Geometry check sheet. Reference: the model listing, model coordinates, mm. Face numbers are marked on the shaded views. A direction names the side the tool comes from. Give positions to 0.01 mm unless a question says otherwise; leave off trailing zeros. Loops run counter-clockwise (first coordinate to the right, second up) from the corner with the lowest first, then second, coordinate; pieces in that order, holes last. Notation, with made-up numbers: (7.25, 55.5) -> (21.25, 55.5) arc R27 cw to (21.25, 89.5) -> close; hole circle Ø6 at (57.25, 34.25). An arc over 180 degrees is marked (long way). Write each question's results on one line, items separated by ' | '. Start each with the question number.
1) Draft check along Z on the marked faces 1, 2 and 3. Enter one of: pulls with the +Z half, pulls with the -Z half, needs draft (parallel to the pull), parting line crosses it, or undercut.
2) Scan lines: line 1 (Z direction, x = 0.6, y = 0); line 2 (Z direction, x = -11.5, y = -7.5); line 3 (Y direction, x = -6, z = 7.25). Record each from-to range of solid material in increasing order. Write a range as from..to.
3) Set-up check for the marked faces 4, 5 and 6: record each of +Z, -Z, +X, -X, +Y, -Y from which the full face is reachable in a straight line by a thin tool's end or side.
4) Depth check by flat-ended pin: pin 1 (3 mm diameter, centred on x = -8, z = -6, fed in from +Y); pin 2 (12 mm diameter, centred on x = -2.5, y = 1.5, fed in from +Z); pin 3 (7.5 mm diameter, centred on x = -14.5, y = 3.5, fed in from -Z); pin 4 (7.5 mm diameter, centred on x = -13.5, y = 1.5, fed in from +Z). Enter the tip coordinate at first touch or a pass-through.
5) Sectioned sample at B-B on x = -12.5. Record the cut outline in (y, z), then the cut area to 3 significant figures.
6) Sectioned sample at D-D on x = -19. Record the cut outline in (y, z), then the cut area to 3 significant figures.
7) Sectioned sample at C-C on x = 6.5. Record the cut outline in (y, z), then the cut area to 3 significant figures.
8) Sectioned sample at A-A on z = 0. Record the cut outline in (x, y).
```python
from build123d import *

# Parameters (mm, degrees)
CROQUIS1_ONE_SIDE_W     = 3.003658151
CROQUIS1_ONE_SIDE_H     = 0.614983514
CROQUIS2_W              = 2.5
CROQUIS2_H              = 25
SALIENTE_EXTRUIR1_DEPTH = 25
CORTAR_EXTRUIR1_DEPTH   = 25


with BuildPart() as part:
    # Croquis1 one side → Revolución1 (revolve)
    with BuildSketch(Plane.XY, mode=Mode.PRIVATE) as revoluci_n1_sk:
        Polygon((-3.75, 15), (-3.75, 0), (3.75, 0), (8.75, 0), (8.75, 5), (3.75, 5), (3.75, 15), (1.503658151, 15), (0.751829076, 13.697793843), (-0.751829076, 13.697793843), (-1.503658151, 15), align=None)
        with Locations((0.001829075, 4.692508243)):
            Rectangle(CROQUIS1_ONE_SIDE_W, CROQUIS1_ONE_SIDE_H, mode=Mode.SUBTRACT)
    revolve(revoluci_n1_sk.sketch.rotate(Axis((-10.104371621, 0, 0), (1, 0, 0)), 180), axis=Axis((-10.104371621, 0, 0), (1, 0, 0)))

    # Croquis2 → Saliente-Extruir1 (add)
    with BuildSketch(Plane.ZY.offset(3.75)):
        with Locations((-6.75, 0)):
            Rectangle(CROQUIS2_W, CROQUIS2_H)
        with Locations((6.75, 0)):
            Rectangle(CROQUIS2_W, CROQUIS2_H)
    extrude(amount=SALIENTE_EXTRUIR1_DEPTH)

    # Croquis3 → Cortar-Extruir1 (cut)
    with BuildSketch(Plane.XY.offset(8)):
        with BuildLine():
            Line((-16.469719797, 12.5), (-28.75, 12.5))
            Line((-28.75, 12.5), (-28.75, 0.219719797))
            ThreePointArc((-28.75, 0.219719797), (-25.090200133, 8.840200133), (-16.469719797, 12.5))
        make_face()
        with BuildLine():
            Line((-28.75, -0.219719797), (-28.75, -12.5))
            Line((-28.75, -12.5), (-16.469719797, -12.5))
            ThreePointArc((-16.469719797, -12.5), (-25.090200133, -8.840200133), (-28.75, -0.219719797))
        make_face()
        with BuildLine():
            ThreePointArc((-11.25, 0), (-12.714466094, 3.535533906), (-16.25, 5))
            Line((-16.25, 5), (-16.25, -5))
            ThreePointArc((-16.25, -5), (-12.714466094, -3.535533906), (-11.25, 0))
        make_face()
        with BuildLine():
            Line((-16.25, -5), (-16.25, 5))
            ThreePointArc((-16.25, 5), (-21.25, 0), (-16.25, -5))
        make_face()
    extrude(amount=-CORTAR_EXTRUIR1_DEPTH, mode=Mode.SUBTRACT)


solid = part.part
```
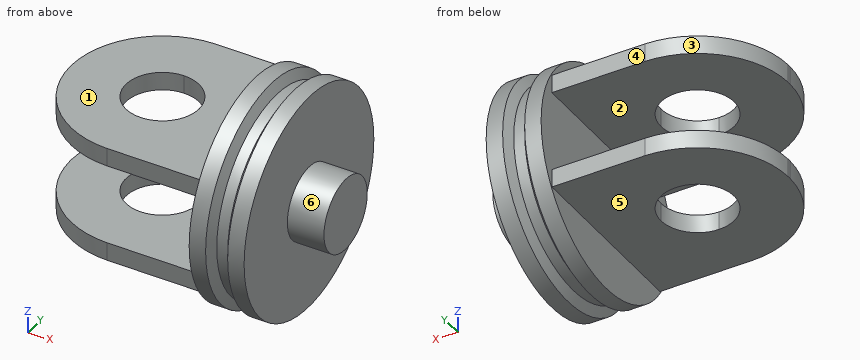
Result:
1) face 1: pulls with the +Z half | face 2: undercut | face 3: needs draft
2) line 1: -13.7..-5, -4.39..4.39, 5..13.7 | line 2: -8..-5.5, 5.5..8 | line 3: -12.5..12.5
3) face 4: +Z, -Z, -X, +Y | face 5: -Z, -X, +Y, -Y | face 6: +X
4) pin 1: y = 12.5 | pin 2: z = 15 | pin 3: z = -8 | pin 4: z = 8
5) outline: (-12.5, -8) -> (-3.31, -8) -> (-3.31, -5.5) -> (-12.5, -5.5) -> close; (-12.5, 5.5) -> (-3.31, 5.5) -> (-3.31, 8) -> (-12.5, 8) -> close; (3.31, -8) -> (12.5, -8) -> (12.5, -5.5) -> (3.31, -5.5) -> close; (3.31, 5.5) -> (12.5, 5.5) -> (12.5, 8) -> (3.31, 8) -> close | area: 91.9 mm^2
6) outline: (-12.2, -8) -> (-4.18, -8) -> (-4.18, -5.5) -> (-12.2, -5.5) -> close; (-12.2, 5.5) -> (-4.18, 5.5) -> (-4.18, 8) -> (-12.2, 8) -> close; (4.18, -8) -> (12.2, -8) -> (12.2, -5.5) -> (4.18, -5.5) -> close; (4.18, 5.5) -> (12.2, 5.5) -> (12.2, 8) -> (4.18, 8) -> close | area: 80.2 mm^2
7) outline: circle Ø10 at (0, 0) | area: 78.5 mm^2
8) outline: (-3.75, -15) -> (-1.5, -15) -> (-0.75, -13.7) -> (0.75, -13.7) -> (1.5, -15) -> (3.75, -15) -> (3.75, -5) -> (8.75, -5) -> (8.75, 5) -> (3.75, 5) -> (3.75, 15) -> (1.5, 15) -> (0.75, 13.7) -> (-0.75, 13.7) -> (-1.5, 15) -> (-3.75, 15) -> close; hole (-1.5, -5) -> (1.5, -5) -> (1.5, -4.39) -> (-1.5, -4.39) -> close; hole (-1.5, 4.39) -> (1.5, 4.39) -> (1.5, 5) -> (-1.5, 5) -> close
